from build123d import *

# Parameters (mm, degrees)
SKETCH2_W           = 3.5
SKETCH2_H           = 9.5
BOSS_EXTRUDE1_DEPTH = 0.3
SKETCH3_W           = 0.3
SKETCH3_H           = 0.1
BOSS_EXTRUDE2_DEPTH = 20


with BuildPart() as part:
    # Sketch2 → Boss-Extrude1 (new body)
    with BuildSketch(Plane(origin=(0, 0, 0), x_dir=(1, 0, 0), z_dir=(0, 1, 0))):
        Rectangle(SKETCH2_W, SKETCH2_H)
    extrude(amount=BOSS_EXTRUDE1_DEPTH)

    # Sketch3 → Boss-Extrude2 (add)
    with BuildSketch(Plane.XY.offset(4.75)):
        with Locations((-0.75, 0.15)):
            Rectangle(SKETCH3_W, SKETCH3_H)
        with Locations((0.6, 0.15)):
            Rectangle(SKETCH3_W, SKETCH3_H)
    extrude(amount=BOSS_EXTRUDE2_DEPTH)


solid = part.part
Work out the finished part from the listing and answer in its coordinate system (mm). Round coordinates to 2 decimals unless told otherwise and drop trailing zeros. Loops run counter-clockwise (first coordinate to the right, second up) from the corner with the lowest first, then second, coordinate; pieces in that order, holes last. Notation, with made-up numbers: M 33.5,-3.5 L 53.5,-3.5 A27 ccw 53.5,19.5 Z; hole C 60.5,8.5 d3. An arc over 180 degrees is marked long. One line per question, with ' | ' between items. Start each with the question number.
(1) A cutting plane is placed at A-A on z = 10.25. Write down the section's boundary in (x, y).
(2) A cutting plane is placed at B-B on y = 0.15. Write down the section's boundary in (x, z).
(3) A cutting plane is placed at C-C on x = 1.35. Write down the section's boundary in (y, z), plus the area to 3 significant figures.
(4) Find the intervals of material crossed by line 1 (Z direction, x = -1.25, y = 0.15), in increasing order.
Geometry check:
1) outline: M -0.9,0.1 L -0.6,0.1 L -0.6,0.2 L -0.9,0.2 Z; M 0.45,0.1 L 0.75,0.1 L 0.75,0.2 L 0.45,0.2 Z
2) outline: M -1.75,-4.75 L 1.75,-4.75 L 1.75,4.75 L 0.75,4.75 L 0.75,24.75 L 0.45,24.75 L 0.45,4.75 L -0.6,4.75 L -0.6,24.75 L -0.9,24.75 L -0.9,4.75 L -1.75,4.75 Z
3) outline: M 0,-4.75 L 0.3,-4.75 L 0.3,4.75 L 0,4.75 Z | area: 2.85 mm²
4) line 1: z = -4.75 to 4.75
